For this review, take the finished solid that the model builds, in its own axes (mm). Face numbers are marked on the shaded views. A direction names the side the tool comes from. Coordinates: 2 decimals unless noted, no trailing zeros. Loops run counter-clockwise (first coordinate to the right, second up) from the corner with the lowest first, then second, coordinate; pieces in that order, holes last. Notation, with made-up numbers: M 10.25,68 L 63.25,68 A8 ccw 63.25,82 Z; hole C -38.75,16 d5. An arc over 180 degrees is marked long. Answer as a JSON object with one key per item and string values. Group by question number.
Item 1: Add section D-D (x = -1.25). State the section outline as (y, z) points (3 decimals).
Item 2: Add section C-C (y = 1). State the section outline as (x, z) points, then the cut area to 3 significant figures.
Item 3: Insertion check: pin 1 (1.5 mm diameter, centred on y = 2, z = 24.5, fed in from +X). The pin has a flat end and moves straight along its axis. Give the tip position at first contact, or say it passes through.
Item 4: Wall thickness on L1, parallel to X at y = 2, z = 10.5; L2, parallel to Y at x = -1, z = 18.75; L3, parallel to Y at x = 2.75, z = 17.75: over which ranges is each line inside the solid? List them lowest first. Write a range as from..to.
Item 5: Add section A-A (x = 0). State the section outline as (y, z) points (3 decimals).
Item 6: Add section B-B (z = 21.5). State the section outline as (x, y) points (3 decimals).
Item 7: Tool access review of the marked faces 1 and 2: name each direction out of +Z, -Z, +X, -X, +Y, -Y from which nothing blocks a thin tool from reaching the whole face with its end or side.
from build123d import *

# Parameters (mm, degrees)
BOSS_EXTRUDE1_DEPTH = 29.4
CUT_EXTRUDE1_DEPTH  = 15


with BuildPart() as part:
    # Sketch1 → Boss-Extrude1 (new body)
    with BuildSketch(Plane.XY):
        with BuildLine():
            Line((1.710263138, 2.675), (0, 2.675))
            Line((0, 2.675), (-1.710263138, 2.675))
            ThreePointArc((-1.710263138, 2.675), (-1.524883526, -2.784843843), (3.175, 0))
            ThreePointArc((3.175, 0), (2.784843843, 1.524883526), (1.710263138, 2.675))
        make_face()
        with BuildLine():
            Line((-1.710263138, 2.675), (0, 2.675))
            Line((0, 2.675), (1.710263138, 2.675))
            ThreePointArc((1.710263138, 2.675), (0, 3.175), (-1.710263138, 2.675))
        make_face()
    extrude(amount=BOSS_EXTRUDE1_DEPTH)

    # Sketch1_3 → Cut-Extrude1 (cut)
    with BuildSketch(Plane.XY):
        with BuildLine():
            Line((-1.710263138, 2.675), (0, 2.675))
            Line((0, 2.675), (1.710263138, 2.675))
            ThreePointArc((1.710263138, 2.675), (0, 3.175), (-1.710263138, 2.675))
        make_face()
    extrude(amount=CUT_EXTRUDE1_DEPTH, mode=Mode.SUBTRACT)


solid = part.part
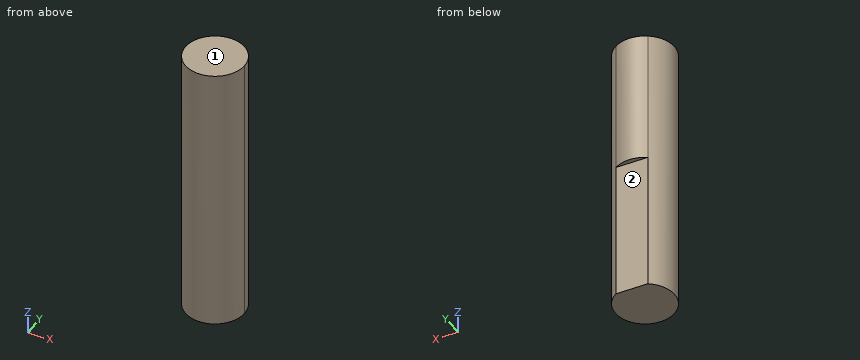
From the geometry:
{
 "1": {"outline": "M -2.919,0 L 2.675,0 L 2.675,15 L 2.919,15 L 2.919,29.4 L -2.919,29.4 Z"},
 "2": {"outline": "M -3.01,0 L 3.01,0 L 3.01,29.4 L -3.01,29.4 Z", "area": "177 mm²"},
 "3": {"pin 1": "stops at x = 2.92"},
 "4": {"L1": "x = -2.47..2.47", "L2": "y = -3.01..3.01", "L3": "y = -1.59..1.59"},
 "5": {"outline": "M -3.175,0 L 2.675,0 L 2.675,15 L 3.175,15 L 3.175,29.4 L -3.175,29.4 Z"},
 "6": {"outline": "C 0,0 d6.35"},
 "7": {"face 1": "+Z, +X, -X, +Y, -Y", "face 2": "-Z, +X, -X, +Y"}
}
